Autodesk Inventor part; units mm, degrees
ref_plane "YZ Plane" through (0, 0, 0) normal (1, 0, 0) x (0, 1, 0)
ref_plane "XZ Plane" through (0, 0, 0) normal (0, 1, 0) x (-1, 0, 0)
ref_plane "XY Plane" through (0, 0, 0) normal (0, 0, 1) x (1, 0, 0)
sketch "Sketch1" plane through (0, 0, 0) normal (0, 0, 1) x (1, 0, 0)
  circle A0 centre (0, 0) radius 3.555
  line L0 (0, 5.7735) -> (5, 2.8868)
  line L1 (5, 2.8868) -> (5, -2.8868)
  line L2 (5, -2.8868) -> (0, -5.7735)
  line L3 (0, -5.7735) -> (-5, -2.8868)
  line L4 (-5, -2.8868) -> (-5, 2.8868)
  line L5 (-5, 2.8868) -> (0, 5.7735)
  circle A1 centre (0.79, 0) radius 2.5
  dimension "d0" = 7.11
  dimension "d2" = 10
  dimension "d3" = 5
  dimension "d4" = 0.79
extrude "Extrusion1" add sketch "Sketch1" along normal blind 6.35 contours A0 | L0 L1 L2 L3 L4 L5
sketch "Sketch2" plane through (0, 0, 6.35) normal (0, 0, 1) x (1, 0, 0)
  circle A0 centre (0.79, 0) radius 2.5
  circle A1 centre (0, 0) radius 3.555
  circle A2 centre (0.79, 0) radius 2.5
  dimension "d7" = 7.11
  dimension "d9" = 5
extrude "Extrusion2" add sketch "Sketch2" along normal blind 2.5
sketch "Sketch3" plane through (5, -2.8868, 0) normal (1, 0, 0) x (0, 0, -1)
  line L0 (0, 5.7735) -> (0, 0)
  line L1 (-6.35, 0) -> (-6.35, 5.7735)
  line L2 (-6.35, 3.8868) -> (0, 3.8868)
  line L3 (0, 1.8868) -> (-6.35, 1.8868)
  line L4 (-6.35, 2.8868) -> (0, 2.8868) construction
  line L5 (-1.966, 2.8868) -> (-1.966, 3.8868) construction
  line L6 (-1.966, 2.8868) -> (-1.966, 1.8868) construction
  dimension "d13" = 2
extrude "Extrusion3" cut sketch "Sketch3" against normal blind 0.25
sketch "Sketch4" plane through (0, 0, 6.35) normal (0, 0, 1) x (1, 0, 0)
  line L0 (3.1264, 5.415) -> (6.2527, 0)
  line L1 (6.2527, 0) -> (3.1264, -5.415)
  line L2 (3.1264, -5.415) -> (-3.1264, -5.415)
  line L3 (-3.1264, -5.415) -> (-6.2527, 0)
  line L4 (-6.2527, 0) -> (-3.1264, 5.415)
  line L5 (-3.1264, 5.415) -> (3.1264, 5.415)
  line L6 (-3.1264, 5.415) -> (0, 7.4304)
  line L7 (0, 7.4304) -> (3.1264, 5.415)
  line L8 (-3.1264, 5.415) -> (-7.0189, 5.2081)
  line L9 (-7.0189, 5.2081) -> (-6.2527, 0)
  line L10 (-6.2527, 0) -> (-7.6169, -4.7381)
  line L11 (-7.6169, -4.7381) -> (-3.1264, -5.415)
  line L12 (-3.1264, -5.415) -> (-0.7756, -8.4436)
  line L13 (-0.7756, -8.4436) -> (3.1264, -5.415)
  line L14 (3.1264, -5.415) -> (7.3563, -3.9182)
  line L15 (7.3563, -3.9182) -> (6.2527, 0)
  line L16 (6.2527, 0) -> (7.7493, 2.746)
  line L17 (7.7493, 2.746) -> (3.1264, 5.415)
  point P0 (0, 0)
  point P1 (0, 0)
  dimension "d16" = 10.83
extrude "Extrusion4" cut sketch "Sketch4" against normal up to surface (6.35 mm away) contours L17 L16 L0 | L5 L6 L7 | L15 L14 L1 | L4 L9 L8 | L13 L12 L2 | L3 L11 L10
properties part number "OpenBuilds_Eccentric_Spacer"
Read the model definition and answer for the solid it produces. Units are mm, in the model's axes. A direction names the side the tool comes from. Round coordinates to 2 decimals unless told otherwise and drop trailing zeros. Loops run counter-clockwise (first coordinate to the right, second up) from the corner with the lowest first, then second, coordinate; pieces in that order, holes last.
Q1. Which of the six approach directions +Z, -Z, +X, -X, +Y, -Y give full straight-line access (tool end or side, diameter ignored) to faces 1 (the face through (0, 5.415, 3)), 2 (the face through (0, 4, 6.35))?
Q2. Section A-A on y = 0 is taken. Write down the section's boundary in (x, z) (3 decimals), and give its area (3 significant figures).
Q3. Each of these flat-tipped pins is pushed along its axis until it touches: pin 1 (3 mm diameter, centred on x = 0.79, y = 0, fed in from -Z); pin 2 (3 mm diameter, centred on x = 4, z = 5, fed in from -Y). Where does it stop, or does it pass through?
Q4. Section B-B on z = 2 is taken. Write down the section's boundary in (x, y) (3 decimals).
Q5. Section C-C on x = 1.75 is taken. Write down the section's boundary in (y, z).
Q6. Section D-D on y = -3 is taken. Write down the section's boundary in (x, z), and give its area (3 significant figures).
Q7. Consider probe 1 along Z at (x, y) = (0, -4); probe 2 along X at (y, z) = (1.5, 2.5); probe 3 along X at (y, z) = (-2, 1). Determine where each line is inside the solid, lowest interval first.
Q8. Determine the mould class of faces 3 (the face through (4.685, 2.715, 3.219)), 4 (the face through (4.694, -2.7, 3.219)), 5 (the face through (0.25, 2.44, 4.36)), 6 (the face through (4.75, 0, 3)) for opening direction Y: released by +Y, released by -Y, zero draft, split by the parting line, or undercut.
Output:
1. face 1: +Z, -Z, +X, -X, +Y
1. face 2: +Z
2. outline: (-5, 0) - (-1.71, 0) - (-1.71, 8.85) - (-3.555, 8.85) - (-3.555, 6.35) - (-5, 6.35) - close; (3.29, 0) - (4.75, 0) - (4.75, 6.35) - (3.555, 6.35) - (3.555, 8.85) - (3.29, 8.85) - close
2. area: 35.4 mm2
3. pin 1: passes through
3. pin 2: stops at y = -4.33
4. outline: (-5, -2.17) - (-4.379, -3.245) - (-0.621, -5.415) - (0.621, -5.415) - (4.379, -3.245) - (5, -2.17) - (5, -1) - (4.75, -1) - (4.75, 1) - (5, 1) - (5, 2.17) - (4.379, 3.245) - (0.621, 5.415) - (-0.621, 5.415) - (-4.379, 3.245) - (-5, 2.17) - close; hole circle Ø5 at (0.79, 0)
5. outline: (-4.76, 0) - (-2.31, 0) - (-2.31, 8.85) - (-3.09, 8.85) - (-3.09, 6.35) - (-4.76, 6.35) - close; (2.31, 0) - (4.76, 0) - (4.76, 6.35) - (3.09, 6.35) - (3.09, 8.85) - (2.31, 8.85) - close
6. outline: (-4.52, 0) - (4.52, 0) - (4.52, 6.35) - (1.91, 6.35) - (1.91, 8.85) - (-1.91, 8.85) - (-1.91, 6.35) - (-4.52, 6.35) - close
6. area: 66.9 mm2
7. probe 1: z = 0 to 6.35
7. probe 2: x = -5 to -1.21, 2.79 to 5
7. probe 3: x = -5 to -0.71, 2.29 to 5
8. face 3: released by +Y
8. face 4: released by -Y
8. face 5: undercut
8. face 6: undercut
